Geometry: final body of the model. Coordinates: model frame, mm. Face numbers are marked on the shaded views. A direction names the side the tool comes from. Give positions to 0.01 mm unless a question says otherwise; leave off trailing zeros. Loops run counter-clockwise (first coordinate to the right, second up) from the corner with the lowest first, then second, coordinate; pieces in that order, holes last. Notation, with made-up numbers: (58, 34) - (95, 34) arc R16 cw to (95, 40) - close; hole circle Ø8 at (64.25, 0.5). An arc over 180 degrees is marked (long way). Use one line per item in the form item = value.
```python
from build123d import *

# Parameters (mm, degrees)
BOSS_EXTRUDE1_DEPTH = 3
SKETCH4_W           = 13
SKETCH4_H           = 3
CUT_EXTRUDE1_DEPTH  = 3
SKETCH5_R           = 1.5
CUT_EXTRUDE2_DEPTH  = 3


with BuildPart() as part:
    # Sketch2 → Boss-Extrude1 (new body)
    with BuildSketch(Plane.XY):
        with BuildLine():
            Line((8.250612211, 16.791600065), (8.250612211, -1.508399935))
            ThreePointArc((8.250612211, -1.508399935), (7.664825773, -2.922613498), (6.250612211, -3.508399935))
            Line((6.250612211, -3.508399935), (-10.749387789, -3.508399935))
            ThreePointArc((-10.749387789, -3.508399935), (-12.163601352, -2.922613498), (-12.749387789, -1.508399935))
            Line((-12.749387789, -1.508399935), (-12.749387789, 21.713833017))
            ThreePointArc((-12.749387789, 21.713833017), (-11.183455157, 24.630917763), (-7.886882979, 24.937740684))
            Line((-7.886882979, 24.937740684), (7.029186388, 18.633833017))
            ThreePointArc((7.029186388, 18.633833017), (7.91751778, 17.896781418), (8.250612211, 16.791600065))
        make_face()
    extrude(amount=BOSS_EXTRUDE1_DEPTH)

    # Sketch4 → Cut-Extrude1 (cut)
    with BuildSketch(Plane.XY.offset(3)):
        with BuildLine():
            Line((-12.749387789, 13.091600065), (-3.749387789, 13.091600065))
            Line((-3.749387789, 13.091600065), (-3.749387789, 16.091600065))
            Line((-3.749387789, 16.091600065), (-10.749387789, 16.091600065))
            ThreePointArc((-10.749387789, 16.091600065), (-12.163601352, 16.677386502), (-12.749387789, 18.091600065))
            Line((-12.749387789, 18.091600065), (-12.749387789, 13.091600065))
        make_face()
        with Locations((-6.249387789, 7.291600065)):
            Rectangle(SKETCH4_W, SKETCH4_H)
        with Locations((-6.249387789, 0.991600065)):
            Rectangle(SKETCH4_W, SKETCH4_H)
    extrude(amount=-CUT_EXTRUDE1_DEPTH, mode=Mode.SUBTRACT)

    # Sketch5 → Cut-Extrude2 (cut)
    with BuildSketch(Plane.XY.offset(3)):
        with Locations((-9.249387789, 21.713833017)):
            Circle(SKETCH5_R)
    extrude(amount=-CUT_EXTRUDE2_DEPTH, mode=Mode.SUBTRACT)


solid = part.part
```
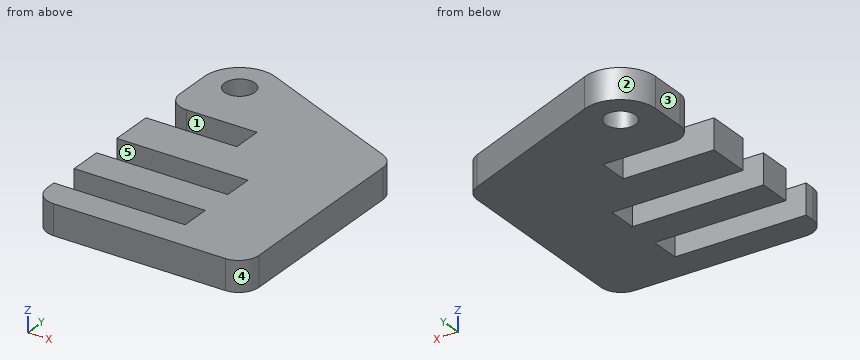
(1) Cut plane A-A (z = 2.05). Return the cut outline in (x, y), plus the area to 3 significant figures.
Solution:
outline = (-12.75, -1.51) arc R2 ccw to (-10.75, -3.51) - (6.25, -3.51) arc R2 ccw to (8.25, -1.51) - (8.25, 16.79) arc R2 ccw to (7.03, 18.63) - (-7.89, 24.94) arc R3.5 ccw to (-12.75, 21.71) - (-12.75, 18.09) arc R2 ccw to (-10.75, 16.09) - (-3.75, 16.09) - (-3.75, 13.09) - (-12.75, 13.09) - (-12.75, 8.79) - (0.25, 8.79) - (0.25, 5.79) - (-12.75, 5.79) - (-12.75, 2.49) - (0.25, 2.49) - (0.25, -0.51) - (-12.75, -0.51) - close; hole circle Ø3 at (-9.25, 21.71)
area = 426 mm2
(2) Cut plane C-C (y = 21). Return the cut outline in (x, z).
Solution:
outline = (-12.75, 0) - (-10.57, 0) - (-10.57, 3) - (-12.75, 3) - close; (-7.93, 0) - (1.43, 0) - (1.43, 3) - (-7.93, 3) - close
(3) Pin query (flat end, axial travel): P1, Ø0.9, axis at y = 1, z = 1.5, coming from the -X side; P2, Ø1.5, axis at x = -6.5, z = 1, coming from the +Y side. Return the tip coordinate at first contact, or that it passes through.
Solution:
P1 = 0.25
P2 = 24.67
(4) Access query for the marked faces 4 and 5. Directions: +Z, -Z, +X, -X, +Y, -Y. A direction counts if a zero-diameter tool reaches every point of the face in a straight line with its end or side. Return the directions, or none.
Solution:
face_4 = +Z, -Z, +X, -Y
face_5 = +Z, -Z, -X
(5) Pull-direction query (Y, two-part tool) for the marked faces 1, 2 and 3; classes: released by +Y, released by -Y, zero draft, split by the parting line, or undercut.
Solution:
face_1 = undercut
face_2 = released by +Y
face_3 = zero draft
(6) Cut plane D-D (y = 7). Return the cut outline in (x, z), plus the area to 3 significant figures.
Solution:
outline = (0.25, 0) - (8.25, 0) - (8.25, 3) - (0.25, 3) - close
area = 24.0 mm2
(7) Material intervals for L1, parallel to Y at x = -8.75, z = 2.2; L2, parallel to Y at x = -11, z = 0.9; L3, parallel to Y at x = -4, z = 1.95, sorted ascending. Write a range as from..to.
Solution:
L1 = -3.51..-0.51, 2.49..5.79, 8.79..13.09, 16.09..20.3, 23.13..25.18
L2 = -3.49..-0.51, 2.49..5.79, 8.79..13.09, 16.11..24.74
L3 = -3.51..-0.51, 2.49..5.79, 8.79..13.09, 16.09..23.3
(8) Cut plane B-B (x = -7). Return the cut outline in (y, z), plus the area to 3 significant figures.
Solution:
outline = (-3.51, 0) - (-0.51, 0) - (-0.51, 3) - (-3.51, 3) - close; (2.49, 0) - (5.79, 0) - (5.79, 3) - (2.49, 3) - close; (8.79, 0) - (13.09, 0) - (13.09, 3) - (8.79, 3) - close; (16.09, 0) - (24.56, 0) - (24.56, 3) - (16.09, 3) - close
area = 57.2 mm2
